from build123d import *

# Parameters (mm, degrees)
BOSS_EXTRUDE1_DEPTH      = 230
BOSS_EXTRUDE1_DEPTH_BACK = 230
SKETCH1_R                = 22.225
SKETCH2_R                = 25.4
SKETCH2_R_2              = 19.05
CUT_EXTRUDE1_DEPTH       = 50
CHAMFER1_SIZE            = 5
CUT_EXTRUDE2_START       = -50
SKETCH3_R                = 25.4
SKETCH3_R_2              = 19.05
CUT_EXTRUDE2_DEPTH       = 50
CHAMFER2_SIZE            = 5


with BuildPart() as part:
    # Sketch1 → Boss-Extrude1 (new, two sides: drawn at the far end of the back side and taken through both)
    with BuildSketch(Plane(origin=(0, 0, 0), x_dir=(1, 0, 0), z_dir=(0, 1, 0)).offset(-BOSS_EXTRUDE1_DEPTH_BACK)):
        with Locations(Location((0, 0, 0), (0, 0, 270))):
            Circle(SKETCH1_R)
    extrude(amount=BOSS_EXTRUDE1_DEPTH + BOSS_EXTRUDE1_DEPTH_BACK)

    # Sketch2 → Cut-Extrude1 (cut)
    with BuildSketch(Plane(origin=(0, 230, 0), x_dir=(1, 0, 0), z_dir=(0, 1, 0))):
        Circle(SKETCH2_R)
        with Locations(Location((0, 0, 0), (0, 0, 270))):
            Circle(SKETCH2_R_2, mode=Mode.SUBTRACT)
    extrude(amount=-CUT_EXTRUDE1_DEPTH, mode=Mode.SUBTRACT)

    # Chamfer1
    # the kernel refuses this chamfer: 5 mm, written as the material it takes off along each edge
    with BuildSketch(Plane(origin=(0, 180, 0), x_dir=(0, 0, 1), z_dir=(1, 0, 0))) as chamfer1_piece_1_section:
        Polygon((22.225, CHAMFER1_SIZE), (22.225 - CHAMFER1_SIZE, 0), (22.225, 0), align=None)
    chamfer1_piece_1 = revolve(axis=Axis((0, 180, 0), (0, -1, 0)), mode=Mode.PRIVATE)
    chamfer1_piece_1 = chamfer1_piece_1 - Plane(origin=(0, 176.598584916, 0), x_dir=(0, 0, 1), z_dir=(0, 1, 0)) * Cylinder(19.05, 89, mode=Mode.PRIVATE)
    add(chamfer1_piece_1, mode=Mode.SUBTRACT)

    # Sketch3 → Cut-Extrude2 (cut)
    with BuildSketch(Plane(origin=(0, -230, 0), x_dir=(-1, 0, 0), z_dir=(0, -1, 0)).offset(CUT_EXTRUDE2_START)):
        Circle(SKETCH3_R)
        with Locations(Location((0, 0, 0), (0, 0, 270))):
            Circle(SKETCH3_R_2, mode=Mode.SUBTRACT)
    extrude(amount=CUT_EXTRUDE2_DEPTH, mode=Mode.SUBTRACT)

    # Chamfer2
    # the kernel refuses this chamfer: 5 mm, written as the material it takes off along each edge
    with BuildSketch(Plane(origin=(0, -180, 0), x_dir=(0, 0, 1), z_dir=(-1, 0, 0))) as chamfer2_piece_1_section:
        Polygon((22.225, CHAMFER2_SIZE), (22.225 - CHAMFER2_SIZE, 0), (22.225, 0), align=None)
    chamfer2_piece_1 = revolve(axis=Axis((0, -180, 0), (0, 1, 0)), mode=Mode.PRIVATE)
    chamfer2_piece_1 = chamfer2_piece_1 - Plane(origin=(0, -176.598584916, 0), x_dir=(0, 0, 1), z_dir=(0, 1, 0)) * Cylinder(19.05, 89, mode=Mode.PRIVATE)
    add(chamfer2_piece_1, mode=Mode.SUBTRACT)


solid = part.part
Can you work these out from the model? Positions are in its coordinate system, mm. A direction names the side the tool comes from. Coordinates: 2 decimals unless noted, no trailing zeros. Loops run counter-clockwise (first coordinate to the right, second up) from the corner with the lowest first, then second, coordinate; pieces in that order, holes last. Notation, with made-up numbers: (26.25, 20) - (83.25, 20) arc R17 cw to (83.25, 35) - close; hole circle Ø5 at (9.5, 22). An arc over 180 degrees is marked (long way). Answer as a JSON object with one key per item and string values. Group by question number.
Item 1: If we section it at B-B (x = 0): List the corners of the cut face in (y, z) for me (3 decimals), plus the area to 3 significant figures.
Item 2: If we section it at C-C (y = 64.5): List the corners of the cut face in (x, z) for me (3 decimals), plus the area to 3 significant figures.
Item 3: If we section it at A-A (z = 0): List the corners of the cut face in (x, y) for me (3 decimals), plus the area to 3 significant figures.
Item 4: For pin 1 (1.5 mm diameter, centred on y = -124, z = 11.5, fed in from -X); pin 2 (3 mm diameter, centred on y = 38.5, z = -2.5, fed in from -X); pin 3 (2 mm diameter, centred on y = 49, z = 3.5, fed in from -X), each with a flat end and sliding along its axis, tell me the tip position at first contact or that it passes through.
Item 5: On a 3-axis mill with a long thin cutter (end or side, diameter ignored), from which of +Z, -Z, +X, -X, +Y, -Y can I reach the whole of each face in a straight line? I mean faces 1 (the face through (-11.59, 204.45, -15.12)), 2 (the face through (-11.59, -203.72, -15.12)), 3 (the face through (18.74, -2.45, 11.95)). Say none if no direction works.
Item 6: If I drill on L1, parallel to Z at x = 15, y = 128; L2, parallel to Z at x = 6, y = 65; L3, parallel to X at y = -109, z = 5, over which ranges is the centre line in solid material (lowest first)? Write a range as from..to.
Returned:
{
 "1": {"outline": "(-230, -19.05) - (-178.175, -19.05) - (-175, -22.225) - (175, -22.225) - (178.175, -19.05) - (230, -19.05) - (230, 19.05) - (178.175, 19.05) - (175, 22.225) - (-175, 22.225) - (-178.175, 19.05) - (-230, 19.05) - close", "area": "19,800 mm²"},
 "2": {"outline": "circle Ø44.45 at (0, 0)", "area": "1,550 mm²"},
 "3": {"outline": "(-22.225, -175) - (-19.05, -178.175) - (-19.05, -230) - (19.05, -230) - (19.05, -178.175) - (22.225, -175) - (22.225, 175) - (19.05, 178.175) - (19.05, 230) - (-19.05, 230) - (-19.05, 178.175) - (-22.225, 175) - close", "area": "19,800 mm²"},
 "4": {"pin 1": "stops at x = -19.45", "pin 2": "stops at x = -22.2", "pin 3": "stops at x = -22.08"},
 "5": {"face 1": "+Y", "face 2": "-Y", "face 3": "+Y, -Y"},
 "6": {"L1": "z = -16.4..16.4", "L2": "z = -21.4..21.4", "L3": "x = -21.66..21.66"}
}
